```python
from build123d import *

# Parameters (mm, degrees)
SKETCH1_R                = 2.5
BOSS_EXTRUDE1_DEPTH      = 55
BOSS_EXTRUDE2_DEPTH      = 0.5
BOSS_EXTRUDE2_DEPTH_BACK = 0.5
SKETCH2_R                = 8.5
BOSS_EXTRUDE3_START      = 2
BOSS_EXTRUDE3_DEPTH      = 2
FILLET1_R                = 2


with BuildPart() as part:
    # Sketch1 → Boss-Extrude1 (new body)
    with BuildSketch(Plane(origin=(0, 0, 0), x_dir=(1, 0, 0), z_dir=(0, 1, 0))):
        with Locations(Location((0, 0, 0), (0, 0, 270))):
            Circle(SKETCH1_R)
    extrude(amount=BOSS_EXTRUDE1_DEPTH)

    # Sketch2 → Boss-Extrude2 (add, two sides: drawn at the far end of the back side and taken through both)
    with BuildSketch(Plane(origin=(0, 0, 0), x_dir=(0, 0, -1), z_dir=(1, 0, 0)).offset(-BOSS_EXTRUDE2_DEPTH_BACK)):
        with Locations((0, 27.5)):
            Circle(SKETCH2_R)
    extrude(amount=BOSS_EXTRUDE2_DEPTH + BOSS_EXTRUDE2_DEPTH_BACK)

    # Sketch3 → Boss-Extrude3 (add)
    with BuildSketch(Plane.XZ.offset(BOSS_EXTRUDE3_START)):
        with BuildLine():
            Line((-2.5, 0), (-2.5, 7.742565285))
            Line((-2.5, 7.742565285), (2.5, 7.742565285))
            Line((2.5, 7.742565285), (2.5, 0))
            ThreePointArc((2.5, 0), (0, -2.5), (-2.5, 0))
        make_face()
    extrude(amount=-BOSS_EXTRUDE3_DEPTH)

    # Fillet1
    fillet1_edges = [part.edges().sort_by_distance(p)[0] for p in [
        (2.5, -1, 7.742565285),
        (-2.5, -1, 7.742565285),
    ]]
    fillet(fillet1_edges, radius=FILLET1_R)


solid = part.part
```
Can you work these out from the model? Positions are in its coordinate system, mm. A direction names the side the tool comes from. Coordinates: 2 decimals unless noted, no trailing zeros. Order: outer loops, then holes, each group sorted by start corner. A loop starts at its lowest first (then second) coordinate and runs counter-clockwise, first axis right, second up.
1. For faces 1 (the face through (0.5, 28, 5)), 2 (the face through (0, -1, 7.743)), 3 (the face through (-0.5, 28, -5)), 4 (the face through (0.5, 28, -5)), 5 (the face through (-0.5, 28, 5)), which set-ups out of +Z, -Z, +X, -X, +Y, -Y let a thin tool reach every point of the face, with its end or its side?
2. Thinking about a two-plate mould opening in Y: for faces 6 (the face through (0, -2, 3)), 7 (the face through (-0.01, 27.65, 8.5)), 8 (the face through (0, 55, 0)), which applies, +Y half, -Y half, draft (parallel to the pull), parting line (faces both ways), or undercut?
3. If we section it at D-D (z = 1.25): Please give me the cut outline in (x, y).
4. If we section it at C-C (y = 38): Please give me the cut outline in (x, z).
5. If we section it at A-A (z = 5): Please give me the cut outline in (x, y), then the cut area to 3 significant figures.
6. If we section it at B-B (x = 0): Please give me the cut outline in (y, z), then the cut area to 3 significant figures.
7. I need wall thicknesses on line 1 (Y direction, x = -1.35, z = 7); line 2 (Z direction, x = -0.45, y = 47); line 3 (X direction, y = 23, z = 2.5). Which ranges of each line are inside material? Lowest first, please.
8. I'm going to push flat-ended pins straight in: pin 1 (3 mm diameter, centred on y = 27.5, z = -4.5, fed in from -X); pin 2 (2.5 mm diameter, centred on x = 0, z = 5, fed in from +Y); pin 3 (10 mm diameter, centred on y = 13, z = 3.5, fed in from -X); pin 4 (2 mm diameter, centred on x = 0, z = -4.5, fed in from -Y). Where does each tip first touch, or does it pass through?
Entries:
1. face 1: +Z, +X, +Y
1. face 2: +Z, +X, -X, -Y
1. face 3: -Z, -X, +Y, -Y
1. face 4: -Z, +X, +Y, -Y
1. face 5: +Z, -X, +Y
2. face 6: -Y half
2. face 7: undercut
2. face 8: +Y half
3. outline: (-2.5, -2) - (2.5, -2) - (2.5, 0) - (2.17, 0) - (2.17, 55) - (-2.17, 55) - (-2.17, 0) - (-2.5, 0) - close
4. outline: circle Ø5 at (0, 0)
5. outline: (-2.5, -2) - (2.5, -2) - (2.5, 0) - (-2.5, 0) - close; (-0.5, 20.63) - (0.5, 20.63) - (0.5, 34.37) - (-0.5, 34.37) - close
5. area: 23.7 mm2
6. outline: (-2, -2.5) - (19.38, -2.5) arc R8.5 ccw to (35.62, -2.5) - (55, -2.5) - (55, 2.5) - (35.62, 2.5) arc R8.5 ccw to (19.38, 2.5) - (0, 2.5) - (0, 7.74) - (-2, 7.74) - close
6. area: 439 mm2
7. line 1: y = -2 to 0
7. line 2: z = -2.46 to 2.46
7. line 3: x = -0.5 to 0.5
8. pin 1: stops at x = -0.5
8. pin 2: stops at y = 35.13
8. pin 3: stops at x = -2.5
8. pin 4: stops at y = 19.75
